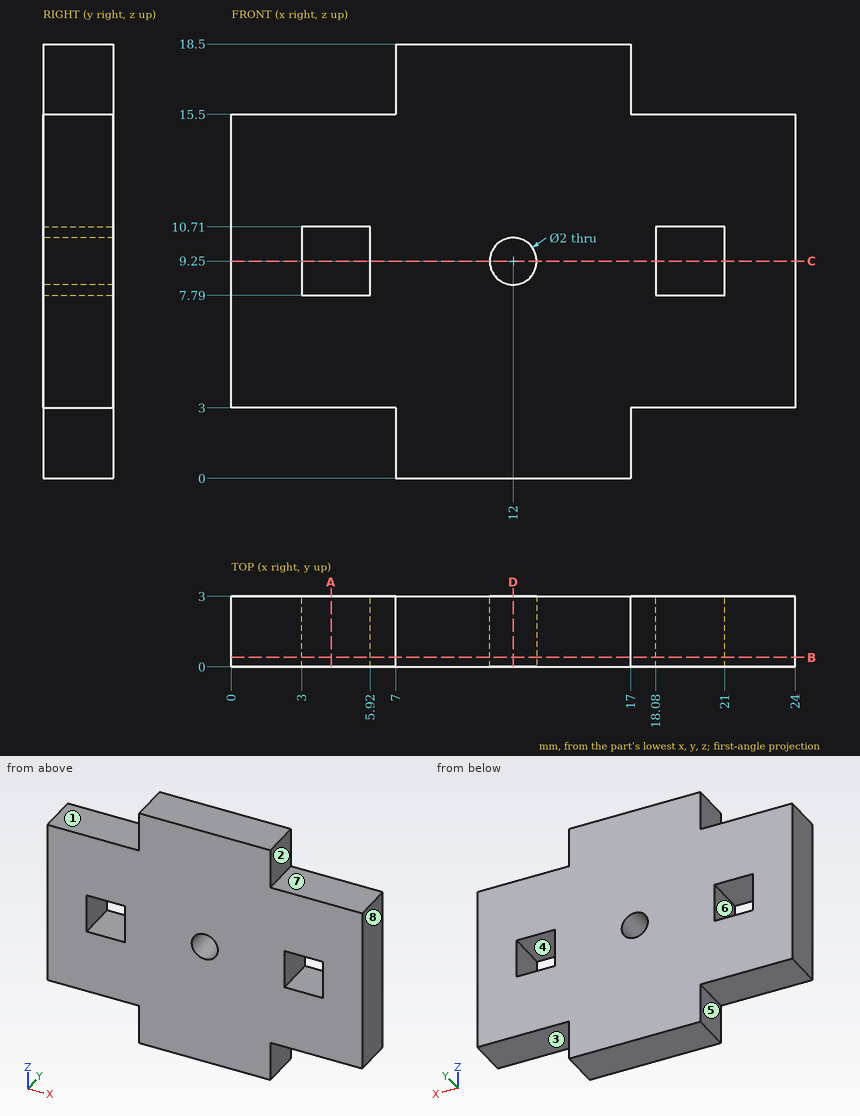
Study the drawing (mm; zero at the part's minimum x, y, z) and answer. A direction names the side the tool comes from. Round coordinates to 2 decimals unless told otherwise and drop trailing zeros. Loops run counter-clockwise (first coordinate to the right, second up) from the corner with the lowest first, then second, coordinate; pieces in that order, holes last.
Q1. Find the intervals of material crossed by line 1 (X direction, y = 0.7, z = 9.25); line 2 (Z direction, x = 12, y = 1.05); line 3 (X direction, y = 0.3, z = 2), in increasing order.
Q2. Section C-C, the plane z = 9.25 is taken. Determine the outline of the cut face in (x, y).
Q3. Section D-D, the plane x = 12 is taken. Determine the outline of the cut face in (y, z), then the cut area to 3 significant figures.
Q4. Which of the six approach directions +Z, -Z, +X, -X, +Y, -Y give full straight-line access (tool end or side, diameter ignored) to the marked faces 1, 2, 3, 4 and 5?
Q5. Given pin 1 Ø0.9 at (x, y) = (4.5, 2) entering from +Z; pin 2 Ø1.5 at (x, y) = (20, 2) entering from -Z; pin 3 Ø0.9 at (y, z) = (2, 1.5) entering from +X, each flat-ended and moving along its own axis, determine where each tip first touches the part or whether it passes through.
Q6. Section A-A, the plane x = 4.25 is taken. Determine the outline of the cut face in (y, z), then the cut area to 3 significant figures.
Q7. For a pull along Z with two mould halves and no side action, classify the marked faces 6, 7 and 8 as released by +Z, released by -Z, zero draft, split by the parting line, or undercut.
Q8. Section B-B, the plane y = 0.4 is taken. Determine the outline of the cut face in (x, z).
Completed:
1. line 1: x = 0 to 3, 5.92 to 11, 13 to 18.08, 21 to 24
1. line 2: z = 0 to 8.25, 10.25 to 18.5
1. line 3: x = 7 to 17
2. outline: (0, 0) - (3, 0) - (3, 3) - (0, 3) - close; (5.92, 0) - (11, 0) - (11, 3) - (5.92, 3) - close; (13, 0) - (18.08, 0) - (18.08, 3) - (13, 3) - close; (21, 0) - (24, 0) - (24, 3) - (21, 3) - close
3. outline: (0, 0) - (3, 0) - (3, 8.25) - (0, 8.25) - close; (0, 10.25) - (3, 10.25) - (3, 18.5) - (0, 18.5) - close
3. area: 49.5 mm2
4. face 1: +Z, -X, +Y, -Y
4. face 2: +Z, +X, +Y, -Y
4. face 3: -Z, +X, +Y, -Y
4. face 4: +Y, -Y
4. face 5: -Z, -X, +Y, -Y
5. pin 1: stops at z = 15.5
5. pin 2: stops at z = 3
5. pin 3: stops at x = 17
6. outline: (0, 3) - (3, 3) - (3, 7.79) - (0, 7.79) - close; (0, 10.71) - (3, 10.71) - (3, 15.5) - (0, 15.5) - close
6. area: 28.7 mm2
7. face 6: undercut
7. face 7: released by +Z
7. face 8: zero draft
8. outline: (0, 3) - (7, 3) - (7, 0) - (17, 0) - (17, 3) - (24, 3) - (24, 15.5) - (17, 15.5) - (17, 18.5) - (7, 18.5) - (7, 15.5) - (0, 15.5) - close; hole (3, 7.79) - (5.92, 7.79) - (5.92, 10.71) - (3, 10.71) - close; hole circle Ø2 at (12, 9.25); hole (18.08, 7.79) - (21, 7.79) - (21, 10.71) - (18.08, 10.71) - close
